Part model, mm, in its own coordinate system. A direction names the side the tool comes from. Give positions to 0.01 mm unless a question says otherwise; leave off trailing zeros. Order: outer loops, then holes, each group sorted by start corner. A loop starts at its lowest first (then second) coordinate and runs counter-clockwise, first axis right, second up. Notation, with made-up numbers: (8.25, 75) - (25.25, 75) arc R19 cw to (25.25, 83) - close; hole circle Ø10 at (-4, 13). An arc over 180 degrees is marked (long way). Use one line per item in the form item = value. Start each with the question number.
1. Pin check, flat tips, straight feed: P1, Ø2, axis at x = 64, z = 6, coming from the -Y side; P2, Ø3, axis at x = 96.5, z = 7, coming from the +Y side; P3, Ø4, axis at x = 199.5, z = 7, coming from the -Y side; P4, Ø0.9, axis at x = 219, y = 0, coming from the -Z side. Stop position of each tip, or through.
2. Pull direction X, two halves, no side cores. Call faces 1 (the face through (147, -149, 0)), 2 (the face through (0, -215, 6)), 3 (the face through (180.809, -142.155, 5.423)): +X half, -X half, draft (parallel to the pull), parting line (faces both ways), or undercut.
3. Band-saw the part on C-C, the plane x = 79. List the corners of the cut face in (y, z), plus the area to 3 significant figures.
4. Band-saw the part on A-A, the plane z = 8.75. State how many separate pieces and enclosed holes the cut face has, plus the area to 3 significant figures.
5. Drill centre lines: line 1 (Y direction, x = 5, z = 5.5); line 2 (X direction, y = -203.5, z = 6); line 3 (X direction, y = 3, z = 5). Where is each one in solid material? Low to high.
6. Tool access for faces 4 (the face through (25, -188.38, 5.58)), 5 (the face through (10, -188, 5)), 6 (the face through (0, -225, 6)): list every direction of +Z, -Z, +X, -X, +Y, -Y with a clear straight run to the whole face (end or side of a thin tool).
7. Band-saw the part on B-B, the plane y = -14. List the corners of the cut face in (x, z), plus the area to 3 significant figures.
from build123d import *

# Parameters (mm, degrees)
F1_DEPTH  = 11
F2_R      = 28.523991
F3_R      = 5
F5_R      = 0.75
F6_DEPTH  = 11.001
F7_R      = 4
F8_DEPTH  = 11.001
F10_DEPTH = 11.001


with BuildPart() as f1:
    # F0 (on Top) → F1 (new body)
    with BuildSketch(Plane.XY):
        with BuildLine():
            ThreePointArc((-59.119348, -199.42142), (-183.034682, -98.804378), (-199.158229, 60))
            Line((-199.158229, 60), (-222.036033, 60))
            ThreePointArc((-222.036033, 60), (0, -230), (222.036033, 60))
            Line((222.036033, 60), (199.158229, 60))
            ThreePointArc((199.158229, 60), (183.034682, -98.804378), (59.119348, -199.42142))
            Line((59.119348, -199.42142), (25, -188))
            Line((25, -188), (0, -188))
            Line((0, -188), (-25, -188))
            Line((-25, -188), (-59.119348, -199.42142))
        make_face()
    extrude(amount=F1_DEPTH)

    # F2
    f2_edges = [f1.edges().sort_by_distance(p)[0] for p in [
        (25, -188, 5.5),
        (-25, -188, 5.5),
    ]]
    fillet(f2_edges, radius=F2_R)

    # F3
    f3_edges = [f1.edges().sort_by_distance(p)[0] for p in [
        (59.119348, -199.42142, 5.5),
        (-59.119348, -199.42142, 5.5),
    ]]
    fillet(f3_edges, radius=F3_R)

    # F5 (on face) → F6 (cut, through all)
    with BuildSketch(Plane.XY.offset(11)):
        with Locations((0, -219)):
            Circle(F5_R)
        with Locations((48.732085, -213.509213)):
            Circle(F5_R)
        with Locations((95.020539, -197.312182)):
            Circle(F5_R)
        with Locations((136.544267, -171.221095)):
            Circle(F5_R)
        with Locations((171.221095, -136.544267)):
            Circle(F5_R)
        with Locations((197.312182, -95.020539)):
            Circle(F5_R)
        with Locations((213.509213, -48.732085)):
            Circle(F5_R)
        with Locations((219, 0)):
            Circle(F5_R)
        with Locations((213.509213, 48.732085)):
            Circle(F5_R)
        with Locations((197.312182, 95.020539)):
            Circle(F5_R)
        with Locations((171.221095, 136.544267)):
            Circle(F5_R)
        with Locations((136.544267, 171.221095)):
            Circle(F5_R)
        with Locations((95.020539, 197.312182)):
            Circle(F5_R)
        with Locations((48.732085, 213.509213)):
            Circle(F5_R)
        with Locations((0, 219)):
            Circle(F5_R)
        with Locations((-48.732085, 213.509213)):
            Circle(F5_R)
        with Locations((-95.020539, 197.312182)):
            Circle(F5_R)
        with Locations((-136.544267, 171.221095)):
            Circle(F5_R)
        with Locations((-171.221095, 136.544267)):
            Circle(F5_R)
        with Locations((-197.312182, 95.020539)):
            Circle(F5_R)
        with Locations((-213.509213, 48.732085)):
            Circle(F5_R)
        with Locations((-219, 0)):
            Circle(F5_R)
        with Locations((-213.509213, -48.732085)):
            Circle(F5_R)
        with Locations((-197.312182, -95.020539)):
            Circle(F5_R)
        with Locations((-171.221095, -136.544267)):
            Circle(F5_R)
        with Locations((-136.544267, -171.221095)):
            Circle(F5_R)
        with Locations((-95.020539, -197.312182)):
            Circle(F5_R)
        with Locations((-48.732085, -213.509213)):
            Circle(F5_R)
        with Locations((-5, -197)):
            Circle(F5_R)
        with Locations((5, -197)):
            Circle(F5_R)
        with Locations((0, -208)):
            Circle(F5_R)
        with Locations((-5, -217)):
            Circle(F5_R)
        with Locations((-25, -207)):
            Circle(F5_R)
        with Locations((5, -217)):
            Circle(F5_R)
        with Locations((25, -207)):
            Circle(F5_R)
    extrude(amount=-F6_DEPTH, mode=Mode.SUBTRACT)

    # F7 (on face) → F8 (cut, through all)
    with BuildSketch(Plane.XY.offset(11)):
        with Locations((-171.221095, -136.544267)):
            Circle(F7_R)
        with Locations((171.221095, -136.544267)):
            Circle(F7_R)
    extrude(amount=-F8_DEPTH, mode=Mode.SUBTRACT)

    # F9 (on face) → F10 (cut, through all)
    with BuildSketch(Plane.XY.offset(11)):
        Polygon((0, -205), (0, -188), (0, 106.196139), (-257.946059, 106.196139), (-257.946059, -251.474887), (0, -251.474887), (0, -211), (-5, -213.082092), (-5, -202.917908), align=None)
    extrude(amount=-F10_DEPTH, mode=Mode.SUBTRACT)


solid = f1.part
From the geometry:
q1.P1 = -221.2
q1.P2 = -183.47
q1.P3 = -117.87
q1.P4 = through
q2.face_1 = draft
q2.face_2 = undercut
q2.face_3 = +X half
q3.outline = (-216.01, 0) - (-192.41, 0) - (-192.41, 11) - (-216.01, 11) - close
q3.area = 260 mm²
q4.separate_pieces = 1
q4.enclosed_holes = 12
q4.area = 9,690 mm²
q5.line_1 = -229.95 to -217.75, -216.25 to -197.75, -196.25 to -188
q5.line_2 = -5 to -3.6, 0 to 107.18
q5.line_3 = 207.98 to 229.98
q6.face_4 = +Z, -Z, +Y
q6.face_5 = +Z, -Z, -X, +Y
q6.face_6 = +Z, -Z, -X, -Y
q7.outline = (207.53, 0) - (229.57, 0) - (229.57, 11) - (207.53, 11) - close
q7.area = 242 mm²
